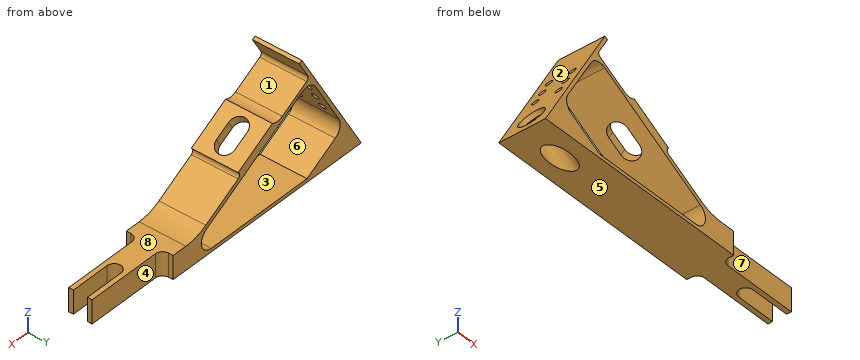
from build123d import *

# Parameters (mm, degrees)
F1_DEPTH  = 10
F4_DEPTH  = 8
F5_R      = 1.5
F6_DEPTH  = 30.83145
F7_R      = 5.5
F7_R_2    = 4.25
F8_DEPTH  = 2
F9_DEPTH  = 112.584302492
F11_DEPTH = 25


with BuildPart() as f1:
    # F0 (on Front) → F1 (new body, symmetric)
    with BuildSketch(Plane.XZ):
        with BuildLine():
            Line((30, 51.9615242271), (0, 0))
            Line((0, 0), (130, 0))
            Line((130, 0), (130, 10))
            Line((130, 10), (88.5384757729, 10))
            ThreePointArc((88.5384757729, 10), (83.3620948709, 10.6814834742), (78.5384757729, 12.6794919243))
            Line((78.5384757729, 12.6794919243), (62.1900542571, 22.1182574873))
            ThreePointArc((62.1900542571, 22.1182574873), (61.4400542571, 23.417295593), (62.1900542571, 24.7163336987))
            Line((62.1900542571, 24.7163336987), (44.8695461814, 34.7163336987))
            ThreePointArc((44.8695461814, 34.7163336987), (42.3695461814, 34.0464607176), (39.8695461814, 34.7163336987))
            Line((39.8695461814, 34.7163336987), (27.5980762114, 41.8012701892))
            ThreePointArc((27.5980762114, 41.8012701892), (26.8991874719, 42.7120797272), (27.0490381057, 43.8503082949))
            Line((27.0490381057, 43.8503082949), (31.2990381057, 51.2115242271))
            Line((31.2990381057, 51.2115242271), (30, 51.9615242271))
        make_face()
        with BuildLine():
            ThreePointArc((13.1291651246, 9.7403810568), (10.7995359932, 12.7764128502), (11.2990381057, 16.5705080757))
            Line((11.2990381057, 16.5705080757), (23.0490381057, 36.9221050646))
            ThreePointArc((23.0490381057, 36.9221050646), (26.0850698991, 39.2517341961), (29.8791651246, 38.7522320835))
            Line((29.8791651246, 38.7522320835), (78.2416697508, 10.8301270189))
            ThreePointArc((78.2416697508, 10.8301270189), (80.5712988822, 5.2059047745), (75.7416697508, 1.5))
            Line((75.7416697508, 1.5), (27.4019237886, 1.5))
            Line((27.4019237886, 1.5), (13.1291651246, 9.7403810568))
        make_face(mode=Mode.SUBTRACT)
    extrude(amount=F1_DEPTH, both=True)

    # F2 (on face) → F4 (cut)
    with BuildSketch(Plane(origin=(26.25, 0, 45.4663336987), x_dir=(0.8660254038, 0, -0.5), z_dir=(0.5, 0, 0.8660254038))):
        with BuildLine():
            ThreePointArc((28, 4), (24, 0), (28, -4))
            Line((28, -4), (35, -4))
            ThreePointArc((35, -4), (39, 0), (35, 4))
            Line((35, 4), (28, 4))
        make_face()
    extrude(amount=-F4_DEPTH, mode=Mode.SUBTRACT)

    # F5 (on offset) → F6 (cut)
    with BuildSketch(Plane(origin=(-21.6506350946, 0, 12.5), x_dir=(0, -1, 0), z_dir=(-0.8660254038, 0, 0.5))):
        with Locations((-5, 39)):
            Circle(F5_R)
        with Locations((5, 39)):
            Circle(F5_R)
        with Locations((-5, 32)):
            Circle(F5_R)
        with Locations((5, 32)):
            Circle(F5_R)
        with Locations((5, 25)):
            Circle(F5_R)
        with Locations((-5, 25)):
            Circle(F5_R)
    extrude(amount=-F6_DEPTH, mode=Mode.SUBTRACT)

    # F7 (on face) → F8 (cut)
    with BuildSketch(Plane(origin=(0, 0, 0), x_dir=(0, -1, 0), z_dir=(-0.8660254038, 0, 0.5))):
        with Locations((0, 9.5)):
            Circle(F7_R)
        with Locations((0, 9.5)):
            Circle(F7_R_2, mode=Mode.SUBTRACT)
    extrude(amount=-F8_DEPTH, mode=Mode.SUBTRACT)

    # F9 (cut, through all): a face of the model
    f9_faces = [f1.faces().sort_by_distance(p)[0] for p in [
        (4.75, 0, 8.227241336),
    ]]
    extrude(f9_faces, amount=-F9_DEPTH, mode=Mode.SUBTRACT)

    # F10 (on face) → F11 (cut)
    with BuildSketch(Plane.XY.offset(10)):
        with BuildLine():
            ThreePointArc((95, 8), (95.8786796564, 5.8786796564), (98, 5))
            Line((98, 5), (130, 5))
            Line((130, 5), (130, 10))
            Line((130, 10), (95, 10))
            Line((95, 10), (95, 8))
        make_face()
        with BuildLine():
            Line((130, -3), (130, 3))
            Line((130, 3), (113, 3))
            ThreePointArc((113, 3), (110, 0), (113, -3))
            Line((113, -3), (130, -3))
        make_face()
        with BuildLine():
            Line((130, -10), (130, -5))
            Line((130, -5), (98, -5))
            ThreePointArc((98, -5), (95.8786796564, -5.8786796564), (95, -8))
            Line((95, -8), (95, -10))
            Line((95, -10), (130, -10))
        make_face()
    extrude(amount=-F11_DEPTH, mode=Mode.SUBTRACT)


solid = f1.part
Design review of the part built by this model. Coordinates are the model's own, in mm. Face numbers are marked on the shaded views. A direction names the side the tool comes from. Round coordinates to 2 decimals unless told otherwise and drop trailing zeros. Write each loop counter-clockwise with the first axis right and the second up, starting at its lowest first coordinate (ties: lowest second). Pieces come first, ordered by that corner, then holes. Notation, with made-up numbers: (1.5, 37.5) -> (42.5, 37.5) arc R22 ccw to (42.5, 44.5) -> close; hole circle Ø6 at (78.5, -20.5). An arc over 180 degrees is marked (long way). One line per item, written item: value. Start each with the question number.
Q1. Insertion check: P1, Ø3, axis at x = 117.5, z = 3, coming from the -Y side; P2, Ø2, axis at y = 9.5, z = 5, coming from the +X side; P3, Ø1, axis at x = 14, y = 7, coming from the +Z side. Each pin has a flat end and moves straight along its axis. Give the tip position at first contact, or say it passes through.
Q2. Tool access review of the marked faces 5, 6, 7 and 8: name each direction out of +Z, -Z, +X, -X, +Y, -Y from which nothing blocks a thin tool from reaching the whole face with its end or side.
Q3. Add section A-A (x = 120.5). Give the boundary of the cut face in (y, z), then the cut area to 3 significant figures.
Q4. Add section B-B (x = 74.5). Give the boundary of the cut face in (y, z), then the cut area to 3 significant figures.
Q5. To check wall thickness, follow probe 1 along Z at (x, y) = (28.5, 5.75); probe 2 along X at (y, z) = (7.25, 4); probe 3 along X at (y, z) = (-8.75, 5.5). State the ranges of each line that lie inside material, in increasing order.
Q6. The part is to be moulded in two halves that separate along Z. For the marked faces 1, 2, 3 and 4, say which applies: pulls with the +Z half, pulls with the -Z half, needs draft (parallel to the pull), parting line crosses it, or undercut.
Response:
1. P1: stops at y = -5
1. P2: stops at x = 95
1. P3: stops at z = 25.11
2. face 5: -Z, +X, -X, +Y, -Y
2. face 6: +Y, -Y
2. face 7: +Z, -Z, +X, -Y
2. face 8: +Z, +X, +Y, -Y
3. outline: (-5, 0) -> (-3, 0) -> (-3, 10) -> (-5, 10) -> close; (3, 0) -> (5, 0) -> (5, 10) -> (3, 10) -> close
3. area: 40.0 mm^2
4. outline: (-10, 0) -> (10, 0) -> (10, 1.5) -> (-10, 1.5) -> close; (-10, 12.99) -> (10, 12.99) -> (10, 15.01) -> (-10, 15.01) -> close
4. area: 70.4 mm^2
5. probe 1: z = 0 to 1.5, 39.29 to 41.28, 46.36 to 49.36
5. probe 2: x = 2.31 to 23.07, 80.07 to 95.1
5. probe 3: x = 3.18 to 20.47, 80.64 to 95
6. face 1: undercut
6. face 2: pulls with the +Z half
6. face 3: undercut
6. face 4: needs draft
